Autodesk Fusion 360 part; units mm, degrees
sketch "MainRest" plane through (0, 0, 0) normal (0, 1, 0) x (1, 0, 0)
  circle A0 centre (0, 0) radius 36 construction
  line L0 (27, 30) -> (-27, 30)
  line L1 (-30, 27) -> (-30, -27)
  line L2 (-27, -30) -> (27, -30)
  line L3 (30, -27) -> (30, 27)
  line L4 (30, 30) -> (-30, -30) construction
  line L5 (-30, 30) -> (30, -30) construction
  circle A1 centre (0, 0) radius 22
  arc A2 (-27, 30) -> (-30, 27) centre (-27, 27) ccw
  arc A3 (27, -30) -> (30, -27) centre (27, -27) ccw
  arc A4 (-30, -27) -> (-27, -30) centre (-27, -27) ccw
  arc A5 (30, 27) -> (27, 30) centre (27, 27) ccw
  dimension "d3" = 72
  dimension "d4" = 60
  dimension "d5" = 60
  dimension "d8" = 44
  dimension "d9" = 3
extrude "Extrude1" add sketch "MainRest" along normal blind 1.2
ref_plane "WorkPlane1" through (-15.5563, 1.9245, -15.5563) normal (0.7071, 0, 0.7071) x (-0.7071, 0, 0.7071)
ref_plane "WorkPlane2" through (15.5563, 0.9394, 15.5563) normal (-0.7071, 0, -0.7071) x (0.7071, 0, -0.7071)
sketch "SensorHolder" plane through (0, 0, 0) normal (0, -1, 0) x (1, 0, 0)
  circle A0 centre (0, 0) radius 22
  arc A1 (27, -30) -> (30, -27) centre (27, -27) ccw
  line L0 (30, -27) -> (30, 27)
  arc A2 (30, 27) -> (27, 30) centre (27, 27) ccw
  line L1 (27, 30) -> (-27, 30)
  arc A3 (-27, 30) -> (-30, 27) centre (-27, 27) ccw
  line L2 (-30, 27) -> (-30, -27)
  arc A4 (-30, -27) -> (-27, -30) centre (-27, -27) ccw
  line L3 (-27, -30) -> (27, -30)
  line L4 (10.8437, -41.9563) -> (-41.9563, 10.8437) construction
  circle A5 centre (0, 0) radius 22 construction
  arc A6 (-29.1233, -20.3743) -> (-29.4263, -20.7386) centre (-26.9042, -22.5282) ccw
  circle A7 centre (0, 0) radius 36
  line L5 (-19.0919, -12.0208) -> (-12.0208, -19.0919) construction
  line L6 (-12.0208, -19.0919) -> (-20.5061, -27.5772) construction
  line L7 (-20.5061, -27.5772) -> (-27.5772, -20.5061) construction
  line L8 (-27.5772, -20.5061) -> (-19.0919, -12.0208) construction
  line L9 (-20.5061, -27.5772) -> (-12.0208, -19.0919) construction
  line L10 (-27.5772, -20.5061) -> (-19.0919, -12.0208)
  line L11 (-19.0919, -12.0208) -> (-20.5061, -10.6066)
  line L12 (-20.5061, -10.6066) -> (-28.9914, -19.0919)
  line L13 (-28.9914, -19.0919) -> (-27.5772, -20.5061)
  line L14 (-20.5061, -27.5772) -> (-12.0208, -19.0919)
  line L15 (-12.0208, -19.0919) -> (-10.6066, -20.5061)
  line L16 (-10.6066, -20.5061) -> (-19.0919, -28.9914)
  line L17 (-19.0919, -28.9914) -> (-20.5061, -27.5772)
  point P0 (-31.1127, -22.6274)
  dimension "d62" = 10
  dimension "d63" = 12
  dimension "d65" = 2
  dimension "d66" = 2
extrude "Extrude5" add sketch "SensorHolder" along normal blind 20 contours L10 L11 L12 L13 | L14 L15 L16 L17
ref_plane "WorkPlane3" through (0, 1.9245, 0) normal (0.7071, 0, 0.7071) x (-0.7071, 0, 0.7071)
mirror "Mirror1" about plane through (0, 1.9245, 0) normal (0.7071, 0, 0.7071) of "Extrude5"
equation "GutterSquareHoleWidth = 60 mm"
equation "GutterHoleDiameter = 72 mm"
equation "d3 = GutterHoleDiameter"
equation "d4 = GutterSquareHoleWidth"
equation "d5 = GutterSquareHoleWidth"
equation "GolfBallDiameter = 43 mm"
equation "GolfHolePadding = 1 mm"
equation "d8 = GolfBallDiameter + GolfHolePadding"
equation "d9 = SquareCornerRounding"
equation "SquareCornerRounding = 3 mm"
equation "SquareBitThickness = 1.2 mm"
equation "d12 = SquareBitThickness"
equation "SensorHeight = 20 mm"
equation "SensorWidth = 10 mm"
equation "SensorDepth = 8 mm"
equation "SensorRealDepth = 12 mm"
equation "SensorScrewBottomOffset = 3 mm"
equation "SensorScrewHoleDiameter = 4 mm"
equation "InsertDiameter = 4 mm"
equation "InsertHeight = 4 mm"
equation "SensorHolderThickness = 2 mm"
equation "d46 = SensorHeight"
equation "d62 = SensorWidth"
equation "d63 = SensorRealDepth"
equation "d65 = SensorHolderThickness"
equation "d66 = SensorHolderThickness"
Verification items for the finished model (mm, model axes). A direction names the side the tool comes from. Give positions to 0.01 mm unless a question says otherwise; leave off trailing zeros. Write each loop counter-clockwise with the first axis right and the second up, starting at its lowest first coordinate (ties: lowest second). Pieces come first, ordered by that corner, then holes. Notation, with made-up numbers: M 58,86.25 L 79,86.25 A24 ccw 79,108.25 Z; hole C 80,36.5 d5. An arc over 180 degrees is marked long. Put each result on its own line as item: value. Start each with the question number.
1. Scan lines: line 1 along Z through (x, y) = (0, 0.7); line 2 along Y through (x, z) = (15, -18). Record each from-to range of solid material in increasing order. Write a range as [from, to].
2. Set-up check for faces 5 (the face through (19.81, -9.86, 11.3)), 6 (the face through (-29.1, 0.59, 29.14)), 7 (the face through (-19.79, -9.86, -11.32)), 8 (the face through (24.8, -9.9, 14.9)): record each of +Z, -Z, +X, -X, +Y, -Y from which the full face is reachable in a straight line by a thin tool's end or side.
3. Go/stop test with a flat-tipped pin: pin 1 Ø12 at (x, y) = (-15.5, -12.5) entering from -Z. Record where the tip stops, or that it passes through.
4. Section check A-A (x = 0). Record the cut outline in (y, z), and give its area (3 significant figures).
5. Draft check along Z on faces 1 (the face through (16, -20, 24)), 2 (the face through (28.274, -9.86, 19.809)), 3 (the face through (-14.8, -9.9, -24.7)), 4 (the face through (23.275, -9.86, 16.204)). Enter one of: +Z half, -Z half, draft (parallel to the pull), parting line (faces both ways), or undercut.
6. Section check D-D (x = -17). Record the cut outline in (y, z), and give its area (3 significant figures).
7. Section check B-B (y = -1.75). Record the cut outline in (x, z), and give its area (3 significant figures).
8. Section check C-C (z = 0). Record the cut outline in (x, y), and give its area (3 significant figures).
Answer list:
1. line 1: [-30, -22], [22, 30]
1. line 2: [0, 1.2]
2. face 5: -Z, -X, -Y
2. face 6: +Z, -X, +Y, -Y
2. face 7: +Z, +X, -Y
2. face 8: -Z, +X, -Y
3. pin 1: z = -28.99
4. outline: M 0,-30 L 1.2,-30 L 1.2,-22 L 0,-22 Z; M 0,22 L 1.2,22 L 1.2,30 L 0,30 Z
4. area: 19.2 mm2
5. face 1: draft
5. face 2: +Z half
5. face 3: -Z half
5. face 4: undercut
6. outline: M -20,-26.9 L 0,-26.9 L 0,-30 L 1.2,-30 L 1.2,-13.96 L 0,-13.96 L 0,-24.07 L -20,-24.07 Z; M 0,13.96 L 1.2,13.96 L 1.2,30 L 0,30 Z
6. area: 95.1 mm2
7. outline: M -28.99,-19.09 L -27.58,-20.51 L -19.09,-12.02 L -20.51,-10.61 Z; M -20.51,-27.58 L -19.09,-28.99 L -10.61,-20.51 L -12.02,-19.09 Z; M 10.61,20.51 L 12.02,19.09 L 20.51,27.58 L 19.09,28.99 Z; M 19.09,12.02 L 20.51,10.61 L 28.99,19.09 L 27.58,20.51 Z
7. area: 96.0 mm2
8. outline: M -30,0 L -22,0 L -22,1.2 L -30,1.2 Z; M 22,0 L 30,0 L 30,1.2 L 22,1.2 Z
8. area: 19.2 mm2
